CAD build for the part. Positions are in the model's coordinates, mm. Face numbers are marked on the shaded views. A direction names the side the tool comes from. Round coordinates to 2 decimals unless told otherwise and drop trailing zeros. Loops run counter-clockwise (first coordinate to the right, second up) from the corner with the lowest first, then second, coordinate; pieces in that order, holes last. Notation, with made-up numbers: (17, 78) - (38, 78) arc R18 cw to (38, 84) - close; hole circle Ø6 at (40, 84.25). An arc over 180 degrees is marked (long way). Use one line per item in the form item = value.
from build123d import *

# Parameters (mm, degrees)
BOSS_EXTRUDE1_DEPTH = 0.2
BOSS_EXTRUDE2_DEPTH = 0.35
BOSS_EXTRUDE3_DEPTH = 0.5
SKETCH2_W           = 20.858957108
SKETCH2_H           = 10.895771928
BOSS_EXTRUDE4_DEPTH = 1
SKETCH3_W           = 24.214928457
SKETCH3_H           = 14.045107393
SKETCH3_W_2         = 20.858957108
SKETCH3_H_2         = 10.895771928
BOSS_EXTRUDE5_DEPTH = 3.5


with BuildPart() as part:
    # Sketch1 → Boss-Extrude1 (new body)
    with BuildSketch(Plane.XY):
        with BuildLine():
            Line((-3.397107478, 0.09272626), (0.002892522, 0.09272626))
            Line((0.002892522, 0.09272626), (0.002892522, -0.10727374))
            Line((0.002892522, -0.10727374), (-3.397107478, -0.10727374))
            Line((-3.397107478, -0.10727374), (-3.895204827, -0.150851611))
            ThreePointArc((-3.895204827, -0.150851611), (-4.038782699, -0.00727374), (-3.895204827, 0.136304132))
            Line((-3.895204827, 0.136304132), (-3.397107478, 0.09272626))
        make_face()
    extrude(amount=BOSS_EXTRUDE1_DEPTH)

    # Sketch1<4> → Boss-Extrude2 (add)
    with BuildSketch(Plane.XY):
        with BuildLine():
            Line((0.402892522, -0.10727374), (0.402892522, 0.09272626))
            Line((0.402892522, 0.09272626), (0.202892522, 0.09272626))
            Line((0.202892522, 0.09272626), (0.202892522, 1.067220881))
            Line((0.202892522, 1.067220881), (-3.397107478, 1.067220881))
            Line((-3.397107478, 1.067220881), (-3.895204827, 1.110798752))
            ThreePointArc((-3.895204827, 1.110798752), (-4.038782699, 0.967220881), (-3.895204827, 0.82364301))
            Line((-3.895204827, 0.82364301), (-3.397107478, 0.867220881))
            Line((-3.397107478, 0.867220881), (0.002892522, 0.867220881))
            Line((0.002892522, 0.867220881), (0.002892522, 0.09272626))
            Line((0.002892522, 0.09272626), (0.002892522, -0.10727374))
            Line((0.002892522, -0.10727374), (0.002892522, -0.881768361))
            Line((0.002892522, -0.881768361), (-3.397107478, -0.881768361))
            Line((-3.397107478, -0.881768361), (-3.895204827, -0.838190489))
            ThreePointArc((-3.895204827, -0.838190489), (-4.038782699, -0.981768361), (-3.895204827, -1.125346232))
            Line((-3.895204827, -1.125346232), (-3.397107478, -1.081768361))
            Line((-3.397107478, -1.081768361), (0.202892522, -1.081768361))
            Line((0.202892522, -1.081768361), (0.202892522, -0.10727374))
            Line((0.202892522, -0.10727374), (0.402892522, -0.10727374))
        make_face()
    extrude(amount=BOSS_EXTRUDE2_DEPTH)

    # Sketch1<5> → Boss-Extrude3 (add)
    with BuildSketch(Plane.XY):
        with BuildLine():
            Line((1.8, 0.09272626), (0.6, 0.09272626))
            Line((0.6, 0.09272626), (0.6, 1.84272626))
            Line((0.6, 1.84272626), (-3.4, 1.84272626))
            Line((-3.4, 1.84272626), (-3.898097349, 1.886304132))
            ThreePointArc((-3.898097349, 1.886304132), (-4.035149554, 1.744700475), (-3.893545897, 1.607648271))
            Line((-3.893545897, 1.607648271), (-3.397107478, 1.667220881))
            Line((-3.397107478, 1.667220881), (0.402892522, 1.667220881))
            Line((0.402892522, 1.667220881), (0.402892522, -1.681768361))
            Line((0.402892522, -1.681768361), (-3.397107478, -1.681768361))
            Line((-3.397107478, -1.681768361), (-3.893545897, -1.62219575))
            ThreePointArc((-3.893545897, -1.62219575), (-4.035149554, -1.759247955), (-3.898097349, -1.900851611))
            Line((-3.898097349, -1.900851611), (-3.4, -1.85727374))
            Line((-3.4, -1.85727374), (0.6, -1.85727374))
            Line((0.6, -1.85727374), (0.6, -0.10727374))
            Line((0.6, -0.10727374), (2, -0.10727374))
            Line((2, -0.10727374), (2, 2.090619677))
            Line((2, 2.090619677), (2.2, 2.090619677))
            Line((2.2, 2.090619677), (2.2, -2.409380323))
            Line((2.2, -2.409380323), (2.8, -2.409380323))
            Line((2.8, -2.409380323), (2.8, 2.090619677))
            Line((2.8, 2.090619677), (3, 2.090619677))
            Line((3, 2.090619677), (3, -2.409380323))
            Line((3, -2.409380323), (3.6, -2.409380323))
            Line((3.6, -2.409380323), (3.6, 2.090619677))
            Line((3.6, 2.090619677), (3.8, 2.090619677))
            Line((3.8, 2.090619677), (3.8, -2.409380323))
            Line((3.8, -2.409380323), (4.4, -2.409380323))
            Line((4.4, -2.409380323), (4.4, 2.090619677))
            Line((4.4, 2.090619677), (4.6, 2.090619677))
            Line((4.6, 2.090619677), (4.6, -2.409380323))
            Line((4.6, -2.409380323), (5.2, -2.409380323))
            Line((5.2, -2.409380323), (5.2, 2.090619677))
            Line((5.2, 2.090619677), (5.4, 2.090619677))
            Line((5.4, 2.090619677), (5.4, -2.409380323))
            Line((5.4, -2.409380323), (6, -2.409380323))
            Line((6, -2.409380323), (6, 2.090619677))
            Line((6, 2.090619677), (6.2, 2.090619677))
            Line((6.2, 2.090619677), (6.2, -2.409380323))
            Line((6.2, -2.409380323), (6.8, -2.409380323))
            Line((6.8, -2.409380323), (6.8, 2.090619677))
            Line((6.8, 2.090619677), (7, 2.090619677))
            Line((7, 2.090619677), (7, -2.409380323))
            Line((7, -2.409380323), (7.6, -2.409380323))
            Line((7.6, -2.409380323), (7.6, -0.159380323))
            Line((7.6, -0.159380323), (9.6, -0.159380323))
            Line((9.6, -0.159380323), (10.098097349, -0.202958194))
            ThreePointArc((10.098097349, -0.202958194), (10.242728512, -0.058327031), (10.098097349, 0.086304132))
            Line((10.098097349, 0.086304132), (9.6, 0.04272626))
            Line((9.6, 0.04272626), (7.4, 0.04272626))
            Line((7.4, 0.04272626), (7.4, -2.20727374))
            Line((7.4, -2.20727374), (7.2, -2.20727374))
            Line((7.2, -2.20727374), (7.2, 2.29272626))
            Line((7.2, 2.29272626), (6.6, 2.29272626))
            Line((6.6, 2.29272626), (6.6, -2.20727374))
            Line((6.6, -2.20727374), (6.4, -2.20727374))
            Line((6.4, -2.20727374), (6.4, 2.29272626))
            Line((6.4, 2.29272626), (5.8, 2.29272626))
            Line((5.8, 2.29272626), (5.8, -2.20727374))
            Line((5.8, -2.20727374), (5.6, -2.20727374))
            Line((5.6, -2.20727374), (5.6, 2.29272626))
            Line((5.6, 2.29272626), (5, 2.29272626))
            Line((5, 2.29272626), (5, -2.20727374))
            Line((5, -2.20727374), (4.8, -2.20727374))
            Line((4.8, -2.20727374), (4.8, 2.29272626))
            Line((4.8, 2.29272626), (4.2, 2.29272626))
            Line((4.2, 2.29272626), (4.2, -2.20727374))
            Line((4.2, -2.20727374), (4, -2.20727374))
            Line((4, -2.20727374), (4, 2.29272626))
            Line((4, 2.29272626), (3.4, 2.29272626))
            Line((3.4, 2.29272626), (3.4, -2.20727374))
            Line((3.4, -2.20727374), (3.2, -2.20727374))
            Line((3.2, -2.20727374), (3.2, 2.29272626))
            Line((3.2, 2.29272626), (2.6, 2.29272626))
            Line((2.6, 2.29272626), (2.6, -2.20727374))
            Line((2.6, -2.20727374), (2.4, -2.20727374))
            Line((2.4, -2.20727374), (2.4, 2.29272626))
            Line((2.4, 2.29272626), (1.8, 2.29272626))
            Line((1.8, 2.29272626), (1.8, 0.09272626))
        make_face()
    extrude(amount=BOSS_EXTRUDE3_DEPTH)

    # Sketch2 → Boss-Extrude4 (add)
    with BuildSketch(Plane(origin=(0, 0, 0), x_dir=(-1, 0, 0), z_dir=(0, 0, -1))):
        with Locations((-3.109940625, -0.224118245)):
            Rectangle(SKETCH2_W, SKETCH2_H)
    extrude(amount=BOSS_EXTRUDE4_DEPTH)

    # Sketch3 → Boss-Extrude5 (add)
    with BuildSketch(Plane(origin=(0, 0, -1), x_dir=(-1, 0, 0), z_dir=(0, 0, -1))):
        with Locations((-3.177155759, -0.199662359)):
            Rectangle(SKETCH3_W, SKETCH3_H)
        with Locations((-3.109940625, -0.224118245)):
            Rectangle(SKETCH3_W_2, SKETCH3_H_2, mode=Mode.SUBTRACT)
    extrude(amount=-BOSS_EXTRUDE5_DEPTH)


solid = part.part
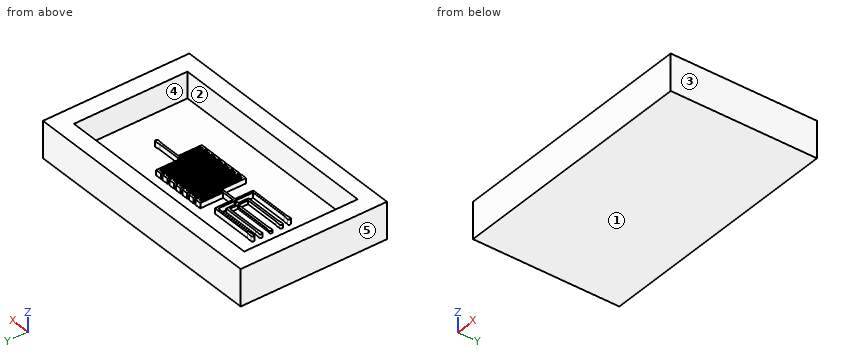
1) Flat gauge pins, fed straight in: pin 1 (5 mm diameter, centred on x = 3.5, y = -0.5, fed in from +Z); pin 2 (5 mm diameter, centred on x = -2.5, y = -4, fed in from +Z). Where does each tip first touch, or does it go through?
Report:
pin_1 = 0.5
pin_2 = 2.5
2) Tool access for the marked faces 1 and 2: list every direction of +Z, -Z, +X, -X, +Y, -Y with a clear straight run to the whole face (end or side of a thin tool).
Report:
face_1 = -Z, +X, -X, +Y, -Y
face_2 = +Z
3) Two-plate mould, pull along X, no slides. Class the marked faces 3, 4 and 5: +X half, -X half, draft (parallel to the pull), parting line (faces both ways), or undercut.
Report:
face_3 = +X half
face_4 = undercut
face_5 = -X half
4) Drill centre lines: probe 1 along Y at (x, z) = (6.5, 0.35); probe 2 along Y at (x, z) = (4.5, 0.35); probe 3 along Y at (x, z) = (8.25, 1.55). Where is each one in solid material? Low to high.
Report:
probe_1 = -7.22 to -5.67, -2.41 to -2.21, 5.22 to 6.82
probe_2 = -7.22 to -5.67, 2.09 to 2.29, 5.22 to 6.82
probe_3 = -7.22 to -5.67, 5.22 to 6.82
5) Slice it at D-D (x = -3). Write the cut outline in (y, z), plus the area to 3 significant figures.
Report:
outline = (-7.22, -1) - (6.82, -1) - (6.82, 2.5) - (5.22, 2.5) - (5.22, 0) - (1.84, 0) - (1.84, 0.5) - (1.67, 0.5) - (1.67, 0) - (1.07, 0) - (1.07, 0.35) - (0.87, 0.35) - (0.87, 0) - (0.09, 0) - (0.09, 0.2) - (-0.11, 0.2) - (-0.11, 0) - (-0.88, 0) - (-0.88, 0.35) - (-1.08, 0.35) - (-1.08, 0) - (-1.68, 0) - (-1.68, 0.5) - (-1.86, 0.5) - (-1.86, 0) - (-5.67, 0) - (-5.67, 2.5) - (-7.22, 2.5) - close
area = 22.3 mm^2
6) Slice it at C-C (y = -3). Write the cut outline in (x, z).
Report:
outline = (-8.93, -1) - (15.28, -1) - (15.28, 2.5) - (13.54, 2.5) - (13.54, 0) - (-7.32, 0) - (-7.32, 2.5) - (-8.93, 2.5) - close
7) Slice it at B-B (x = 8.5). Write the cut outline in (y, z), plus the area to 3 significant figures.
Report:
outline = (-7.22, -1) - (6.82, -1) - (6.82, 2.5) - (5.22, 2.5) - (5.22, 0) - (0.04, 0) - (0.04, 0.5) - (-0.16, 0.5) - (-0.16, 0) - (-5.67, 0) - (-5.67, 2.5) - (-7.22, 2.5) - close
area = 22.0 mm^2
8) Slice it at A-A (z = 2.1). Write the cut outline in (x, y), plus the area to 3 significant figures.
Report:
outline = (-8.93, -7.22) - (15.28, -7.22) - (15.28, 6.82) - (-8.93, 6.82) - close; hole (-7.32, -5.67) - (13.54, -5.67) - (13.54, 5.22) - (-7.32, 5.22) - close
area = 113 mm^2
